Geometry check sheet. Reference: drawing and pictorial views, mm from the part's lowest x, y, z. A direction names the side the tool comes from. Round coordinates to 2 decimals unless told otherwise and drop trailing zeros. Loops run counter-clockwise (first coordinate to the right, second up) from the corner with the lowest first, then second, coordinate; pieces in that order, holes last. Notation, with made-up numbers: (18.25, 55) - (33.25, 55) arc R13 cw to (33.25, 67) - close; hole circle Ø8 at (74.5, 21.25). An arc over 180 degrees is marked (long way). Answer as CSV lines item,"result". Start each with the question number.
1) Depth check by flat-ended pin: P1, Ø0.6, axis at x = 2, y = 6.5, coming from the -Z side (1 decimal); P2, Ø1.5, axis at y = 6.5, z = 2.5, coming from the -X side. Enter the tip coordinate at first touch or a pass-through.
2) Thickness scan on line 1 along Y through (x, z) = (2.2, 0.4); line 2 along Y through (x, z) = (3.25, 1); line 3 along Z through (x, y) = (2.8, 2.25). Record the ranges inside material, lowest first.
3) Access from +Z, -Z, +X, -X, +Y, -Y to the whole of each face (thin tool, end or side, straight path). Record for the marked faces 1 and 2.
4) Cross-section at B-B on y = 2.75. Record the boundary of the cut face in (x, z).
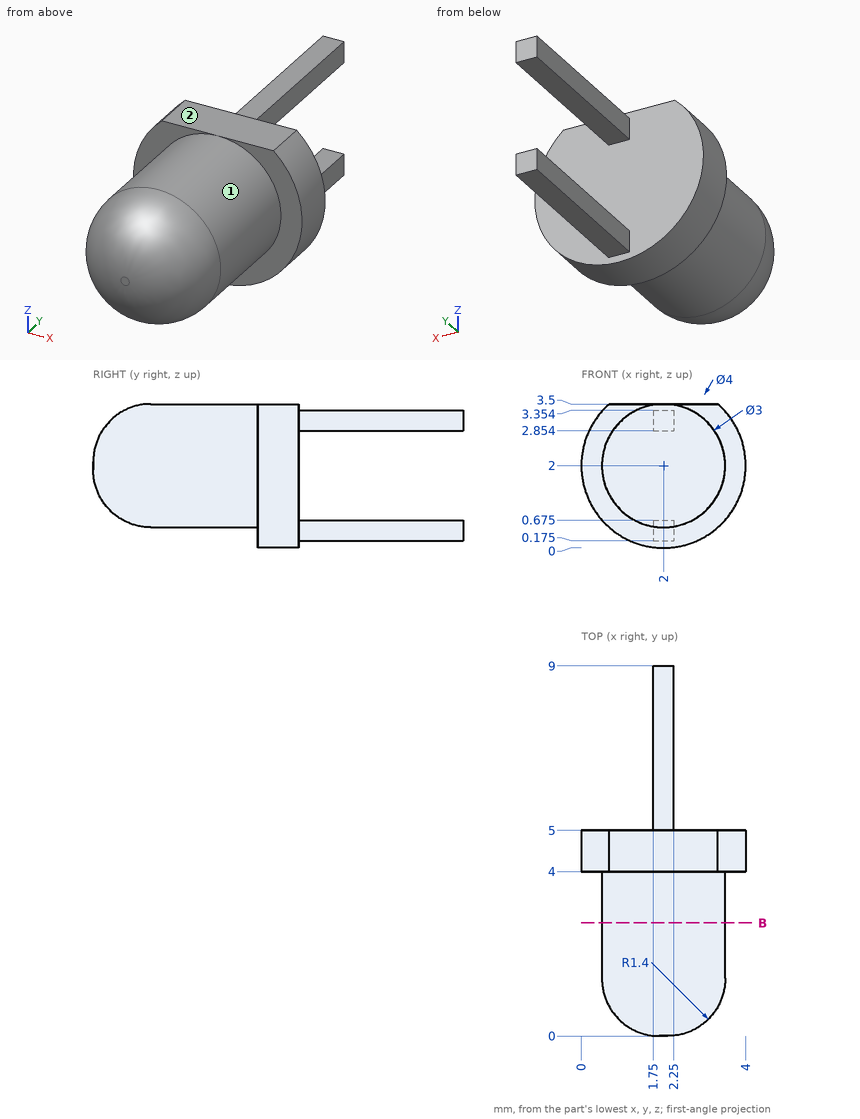
Answer block:
1,P1,"stops at z = 0.2"
1,P2,"stops at x = 1.75"
2,line 1,"y = 4 to 9"
2,line 2,"y = 4 to 5"
2,line 3,"z = 0.73 to 3.27"
3,face 1,"-Y"
3,face 2,"+Z, +X, -X, +Y, -Y"
4,outline,"circle Ø3 at (2, 2)"
